Can you work these out from the model? Positions are in its coordinate system, mm. Coordinates: 2 decimals unless noted, no trailing zeros. Order: outer loops, then holes, each group sorted by start corner. A loop starts at its lowest first (then second) coordinate and runs counter-clockwise, first axis right, second up. Notation, with made-up numbers: M -39,-1 L -10,-1 A10 cw -10,17 Z; hole C 26.5,76.5 d2. An arc over 180 degrees is marked long. Answer as CSV lines item,"result". Start each with the question number.
1. If we section it at A-A (y = 54): List the corners of the cut face in (x, z) for me, plus the area to 3 significant figures.
2. I need wall thicknesses on line 1 along X through (y, z) = (77.5, 4.5); line 2 along Y through (x, z) = (-25.5, 4.3); line 3 along Y through (x, z) = (32, 0.65). Which ranges of each line are inside material? Lowest first, please. Write a range as from..to.
3. If we section it at C-C (y = 30): List the corners of the cut face in (x, z) for me, plus the area to 3 significant figures.
4. If we section it at D-D (z = 4): Give the number of separate pieces and of enclosed holes in the cut face, plus the area to 3 significant figures.
5. Will these pins go through, and if not, where does the flat tip stop? pin 1 (1.7 mm diameter, centred on x = 33, y = -54, fed in from +Z); pin 2 (2.5 mm diameter, centred on x = -32, y = 77.5, fed in from -Z).
6. If we section it at B-B (x = -7): List the corners of the cut face in (y, z) for me.
```python
from build123d import *

# Parameters (mm, degrees)
SKETCH1_W           = 170
SKETCH1_H           = 75
BOSS_EXTRUDE1_DEPTH = 6
SKETCH2_R           = 1.5
CUT_EXTRUDE1_DEPTH  = 94.098066575
CUT_EXTRUDE3_DEPTH  = 3
SKETCH6_W           = 53
SKETCH6_H           = 150
CUT_EXTRUDE4_DEPTH  = 10


with BuildPart() as part:
    # Sketch1 → Boss-Extrude1 (new body)
    with BuildSketch(Plane(origin=(0, 0, 0), x_dir=(0, 1, 0), z_dir=(0, 0, 1))):
        Rectangle(SKETCH1_W, SKETCH1_H)
    extrude(amount=BOSS_EXTRUDE1_DEPTH)

    # Sketch2 → Cut-Extrude1 (cut, through all)
    with BuildSketch(Plane.XY.offset(6)):
        with Locations((-32, 54)):
            Circle(SKETCH2_R)
        with Locations((-32, -54)):
            Circle(SKETCH2_R)
        with Locations((-32, -77.5)):
            Circle(SKETCH2_R)
        with Locations((-32, 77.5)):
            Circle(SKETCH2_R)
        with Locations(Location((32, -77.5, 0), (0, 0, 180))):
            Circle(SKETCH2_R)
        with Locations(Location((32, -54, 0), (0, 0, 180))):
            Circle(SKETCH2_R)
        with Locations(Location((32, 54, 0), (0, 0, 180))):
            Circle(SKETCH2_R)
        with Locations(Location((32, 77.5, 0), (0, 0, 180))):
            Circle(SKETCH2_R)
    extrude(amount=-CUT_EXTRUDE1_DEPTH, mode=Mode.SUBTRACT)

    # Sketch5 → Cut-Extrude3 (cut)
    with BuildSketch(Plane.XY.offset(6)):
        Polygon((-29.15, -55.645448267), (-29.15, -52.354551733), (-32, -50.709103466), (-34.85, -52.354551733), (-34.85, -55.645448267), (-32, -57.290896534), align=None)
        Polygon((32, -57.290896534), (29.15, -55.645448267), (29.15, -52.354551733), (32, -50.709103466), (34.85, -52.354551733), (34.85, -55.645448267), align=None)
        Polygon((-29.15, 55.645448267), (-32, 57.290896534), (-34.85, 55.645448267), (-34.85, 52.354551733), (-32, 50.709103466), (-29.15, 52.354551733), align=None)
        Polygon((29.15, 52.354551733), (29.15, 55.645448267), (32, 57.290896534), (34.85, 55.645448267), (34.85, 52.354551733), (32, 50.709103466), align=None)
    extrude(amount=-CUT_EXTRUDE3_DEPTH, mode=Mode.SUBTRACT)

    # Sketch6 → Cut-Extrude4 (cut)
    with BuildSketch(Plane.XY.offset(6)):
        Rectangle(SKETCH6_W, SKETCH6_H)
    extrude(amount=-CUT_EXTRUDE4_DEPTH, mode=Mode.SUBTRACT)


solid = part.part
```
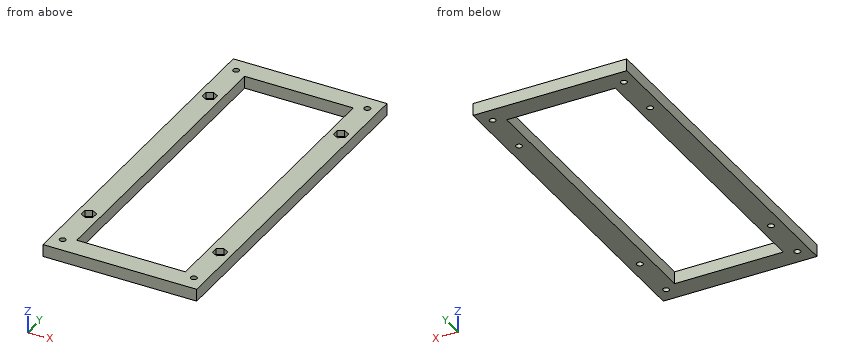
Solved:
1,outline,"M -37.5,0 L -33.5,0 L -33.5,3 L -34.85,3 L -34.85,6 L -37.5,6 Z; M -30.5,0 L -26.5,0 L -26.5,6 L -29.15,6 L -29.15,3 L -30.5,3 Z; M 26.5,0 L 30.5,0 L 30.5,3 L 29.15,3 L 29.15,6 L 26.5,6 Z; M 33.5,0 L 37.5,0 L 37.5,6 L 34.85,6 L 34.85,3 L 33.5,3 Z"
1,area,"79.8 mm²"
2,line 1,"-37.5..-33.5, -30.5..30.5, 33.5..37.5"
2,line 2,"-85..-75, 75..85"
2,line 3,"-85..-79, -76..-55.5, -52.5..52.5, 55.5..76, 79..85"
3,outline,"M -37.5,0 L -26.5,0 L -26.5,6 L -37.5,6 Z; M 26.5,0 L 37.5,0 L 37.5,6 L 26.5,6 Z"
3,area,"132 mm²"
4,separate pieces,"1"
4,enclosed holes,"9"
4,area,"4,660 mm²"
5,pin 1,"z = 3"
5,pin 2,"through"
6,outline,"M -85,0 L -75,0 L -75,6 L -85,6 Z; M 75,0 L 85,0 L 85,6 L 75,6 Z"
